```python
from build123d import *

# Parameters (mm, degrees)
SKETCH_W        = 140
SKETCH_H        = 110
PAD_DEPTH       = 100
SKETCH001_R     = 51
POCKET_DEPTH    = 16.1
SKETCH002_W     = 50
SKETCH002_H     = 7.148574
POCKET001_DEPTH = 16.1
SKETCH003_W     = 140
SKETCH003_H     = 90
POCKET002_DEPTH = 10
POCKET004_DEPTH = 140.001
POCKET005_DEPTH = 140
SKETCH007_R     = 129.123984
POCKET006_DEPTH = 140.001
POCKET007_DEPTH = 140.001
POCKET008_START = -1.5
POCKET008_DEPTH = 5.6
POCKET010_START = -10
POCKET010_DEPTH = 120
POCKET011_DEPTH = 52.16617
POCKET012_START = -20
SKETCH012_R     = 3.5
POCKET012_DEPTH = 30


with BuildPart() as part:
    # Sketch → Pad (new body)
    with BuildSketch(Plane.XY):
        with Locations((70, 55)):
            Rectangle(SKETCH_W, SKETCH_H)
    extrude(amount=PAD_DEPTH)

    # Sketch001 (on Face6 of Pad) → Pocket (cut)
    with BuildSketch(Plane.XY.offset(100)):
        with Locations((69, 61)):
            Circle(SKETCH001_R)
    extrude(amount=-POCKET_DEPTH, mode=Mode.SUBTRACT)

    # Sketch002 (on Face5 of Pocket) → Pocket001 (cut)
    with BuildSketch(Plane.XY.offset(100)):
        with Locations((70, 106.425713)):
            Rectangle(SKETCH002_W, SKETCH002_H)
    extrude(amount=-POCKET001_DEPTH, mode=Mode.SUBTRACT)

    # Sketch003 (on Face5 of Pocket001) → Pocket002 (cut)
    with BuildSketch(Plane.XY.offset(100)):
        with Locations((70, 67)):
            Rectangle(SKETCH003_W, SKETCH003_H)
    extrude(amount=-POCKET002_DEPTH, mode=Mode.SUBTRACT)

    # Sketch005 (on Face2 of Pocket002) → Pocket004 (cut, through all)
    with BuildSketch(Plane(origin=(0, 0, 0), x_dir=(0, -1, 0), z_dir=(-1, 0, 0))):
        Polygon((-18.980759, 100.500006), (7, 85.5), (7, 100.500006), align=None)
    extrude(amount=-POCKET004_DEPTH, mode=Mode.SUBTRACT)

    # Sketch006 (on Face5 of Pocket004) → Pocket005 (cut)
    with BuildSketch(Plane(origin=(0, 0, 0), x_dir=(0, -1, 0), z_dir=(-1, 0, 0))):
        Polygon((-110, 82), (0, 18.491437), (0, 0), (-110, 0), align=None)
    extrude(amount=-POCKET005_DEPTH, mode=Mode.SUBTRACT)

    # Sketch007 (on Face5 of Pocket005) → Pocket006 (cut, through all)
    with BuildSketch(Plane(origin=(0, 0, 0), x_dir=(0, -1, 0), z_dir=(-1, 0, 0))):
        with Locations((-110, -47.123984)):
            Circle(SKETCH007_R)
    extrude(amount=-POCKET006_DEPTH, mode=Mode.SUBTRACT)

    # Sketch008 (on Face5 of Pocket006) → Pocket007 (cut, through all)
    with BuildSketch(Plane(origin=(0, 0, 0), x_dir=(0, -1, 0), z_dir=(-1, 0, 0))):
        Polygon((0, 0), (0, 90), (-29.999995, 38.038473), align=None)
    extrude(amount=-POCKET007_DEPTH, mode=Mode.SUBTRACT)

    # Sketch009 (on Face10 of Pocket007) → Pocket008 (cut)
    with BuildSketch(Plane.XY.offset(90).offset(POCKET008_START)):
        with BuildLine():
            Line((106.36396, 14.264465), (114.142136, 22.042638))
            ThreePointArc((114.142136, 22.042638), (114.727923, 23.456852), (114.142137, 24.871066))
            Line((114.142137, 24.871066), (110.606603, 28.4066))
            ThreePointArc((110.606603, 28.4066), (109.19239, 28.992387), (107.778176, 28.4066))
            Line((107.778176, 28.4066), (100, 20.628427))
            ThreePointArc((100, 20.628427), (99.414214, 19.214214), (100, 17.8))
            Line((100, 17.8), (103.535533, 14.264466))
            ThreePointArc((103.535533, 14.264466), (104.949747, 13.678679), (106.36396, 14.264465))
        make_face()
    extrude(amount=-POCKET008_DEPTH, mode=Mode.SUBTRACT)

    # Sketch010 → Pocket010 (cut)
    with BuildSketch(Plane.YZ.offset(140).offset(POCKET010_START)):
        Polygon((0, 83.24846), (65, 83.24846), (0, 50), align=None)
    extrude(amount=-POCKET010_DEPTH, mode=Mode.SUBTRACT)

    # Sketch011 (on DatumPlane) → Pocket011 (cut, through all)
    with BuildSketch(Plane(origin=(42, -42, 83.24846), x_dir=(0.5, -0.5, 0.707107), z_dir=(0.5, -0.5, -0.707107))):
        with BuildLine():
            Line((8.1, -96.29), (8.1, -85.29))
            ThreePointArc((8.1, -85.29), (7.514214, -83.875786), (6.1, -83.29))
            Line((6.1, -83.29), (1.1, -83.29))
            ThreePointArc((1.1, -83.29), (-0.314214, -83.875786), (-0.9, -85.29))
            Line((-0.9, -85.29), (-0.9, -96.29))
            ThreePointArc((-0.9, -96.29), (-0.314214, -97.704214), (1.1, -98.29))
            Line((1.1, -98.29), (6.1, -98.29))
            ThreePointArc((6.1, -98.29), (7.514214, -97.704214), (8.1, -96.29))
        make_face()
    extrude(amount=POCKET011_DEPTH, mode=Mode.SUBTRACT)

    # Sketch012 (on Face13 of Pocket011) → Pocket012 (cut)
    with BuildSketch(Plane(origin=(0, -38.772597, 67.156073), x_dir=(1, 0, 0), z_dir=(0, -0.5, 0.866025)).offset(POCKET012_START)):
        with Locations((87, 47.5)):
            Circle(SKETCH012_R)
    extrude(amount=-POCKET012_DEPTH, mode=Mode.SUBTRACT)


solid = part.part
```
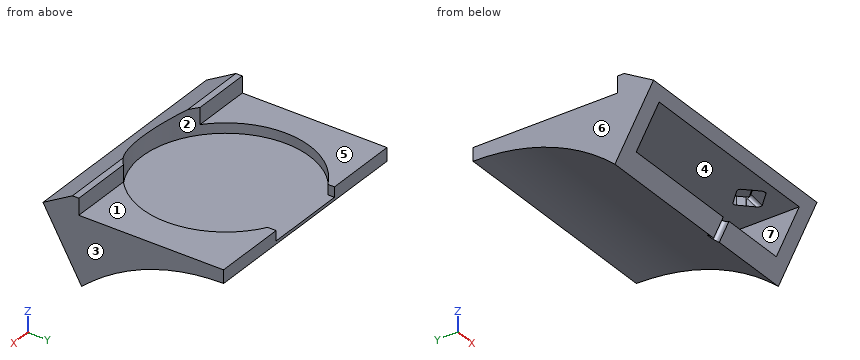
Read the model definition and answer for the solid it produces. Units are mm, in the model's axes. Face numbers are marked on the shaded views. A direction names the side the tool comes from. Coordinates: 2 decimals unless noted, no trailing zeros. Write each loop counter-clockwise with the first axis right and the second up, starting at its lowest first coordinate (ties: lowest second). Pieces come first, ordered by that corner, then holes. Notation, with made-up numbers: (-23.75, 62) -> (6.25, 62) arc R21 cw to (6.25, 86) -> close; hole circle Ø4 at (-30.75, -18). An arc over 180 degrees is marked (long way). Answer as a JSON object with one key per item and string values.
Q1. The part is cut by section A-A on y = 61. Give the vertices of the cut face in (x, z).
The answers:
{"outline": "(0, 72.34) -> (140, 72.34) -> (140, 90) -> (120, 90) -> (120, 83.9) -> (18, 83.9) -> (18, 90) -> (0, 90) -> close; hole (10, 81.2) -> (130, 81.2) -> (130, 83.25) -> (10, 83.25) -> close"}
Q2. Flat-ended cylindrical pins translate along their axes: pin 1 Ø8 at (x, z) = (38.5, 71) entering from -Y; pin 2 Ø5.5 at (y, z) = (106.5, 87) entering from -X; pin 3 Ø12 at (x, y) = (26, 61.5) entering from -Z; pin 4 Ø8 at (x, z) = (88.5, 62.5) entering from -Y. Find the tip coordinate at first contact, or state that the pin passes through.
The answers:
{"pin 1": "stops at y = 33.23", "pin 2": "stops at x = 0", "pin 3": "stops at z = 69.93", "pin 4": "stops at y = 17.83"}
Q3. Determine the mould class of the marked faces 4, 5, 6 and 7 for opening direction Z: pulls with the +Z half, pulls with the -Z half, needs draft (parallel to the pull), parting line crosses it, or undercut.
The answers:
{"face 4": "undercut", "face 5": "pulls with the +Z half", "face 6": "needs draft", "face 7": "undercut"}
Q4. A tool of negligible diameter and unlimited length cuts with its end or side. For the marked faces 1, 2 and 3, from which of +Z, -Z, +X, -X, +Y, -Y can it reach the whole face along a straight path? Write none if from no direction.
The answers:
{"face 1": "+Z, +X, -X, +Y", "face 2": "+Z", "face 3": "+Z, -Z, +X, +Y, -Y"}
Q5. The part is cut by section B-B on x = 73.5. Give the vertices of the cut face in (y, z), then the cut area to 3 significant figures.
The answers:
{"outline": "(0.2, 89.66) -> (3.9, 83.25) -> (65, 83.25) -> (17.83, 59.12) -> (23.71, 48.93) arc R129.12 cw to (110, 82) -> (110, 83.9) -> (10.2, 83.9) -> (10.2, 95.43) -> close", "area": "753 mm2"}
Q6. The part is cut by section C-C on y = 83. Give the vertices of the cut face in (x, z).
The answers:
{"outline": "(0, 79.15) -> (140, 79.15) -> (140, 90) -> (115.01, 90) -> (115.01, 83.9) -> (22.99, 83.9) -> (22.99, 90) -> (0, 90) -> close"}
Q7. The part is cut by section D-D on z = 68. Give the vertices of the cut face in (x, y).
The answers:
{"outline": "(0, 12.7) -> (10, 12.7) -> (10, 35.19) -> (130, 35.19) -> (130, 12.7) -> (140, 12.7) -> (140, 51.52) -> (0, 51.52) -> close"}
Q8. Consider line 1 (X direction, y = 61, z = 88.75); line 2 (X direction, y = 38.5, z = 79); line 3 (Z direction, x = 100.5, y = 60.5). Determine where each line is inside the solid, lowest interval first. Write a range as [from, to].
The answers:
{"line 1": "x = [0, 18], [120, 140]", "line 2": "x = [0, 10], [130, 140]", "line 3": "z = [72.14, 80.95], [83.25, 83.9]"}
